Source: three-view drawing plus pictorial views. Frame: mm from the lowest corner of the part. Coordinates: 2 decimals unless noted, no trailing zeros. Write each loop counter-clockwise with the first axis right and the second up, starting at its lowest first coordinate (ties: lowest second). Pieces come first, ordered by that corner, then holes. Notation, with made-up numbers: (76, -0.5) - (91, -0.5) arc R25 cw to (91, 19.5) - close; hole circle Ø5 at (67, -25.5). An arc over 180 degrees is marked (long way). Answer as a JSON object with one key per item and string values. Group by question number.
Item 1: Section D-D on x = 30.5. Return loops of the section in (y, z), and give its area (3 significant figures).
Item 2: Section C-C on y = 82.5. Return loops of the section in (x, z), and give its area (3 significant figures).
Item 3: Line query: line 1 along Y through (x, z) = (25, 1.65); line 2 along X through (y, z) = (15.5, 1.05); line 3 along X through (y, z) = (81, 2). Output: solid intervals per line, ascending. Write a range as from..to.
Item 4: Section B-B on z = 1.4. Return loops of the section in (x, y), and give its area (3 significant figures).
Item 5: First-contact query: pin 1 Ø3 at (x, y) = (38, 33) entering from -Z; pin 2 Ø1.5 at (y, z) = (86.5, 1) entering from -X; pin 3 Ø1 at (x, z) = (21.5, 3.5) entering from +Y; pin 4 Ø1.3 at (x, z) = (20.5, 1.5) entering from -Y. Flat tips, straight axial feed; report the tip coordinate or a pass-through.
Item 6: Section A-A on x = 25. Return loops of the section in (y, z).
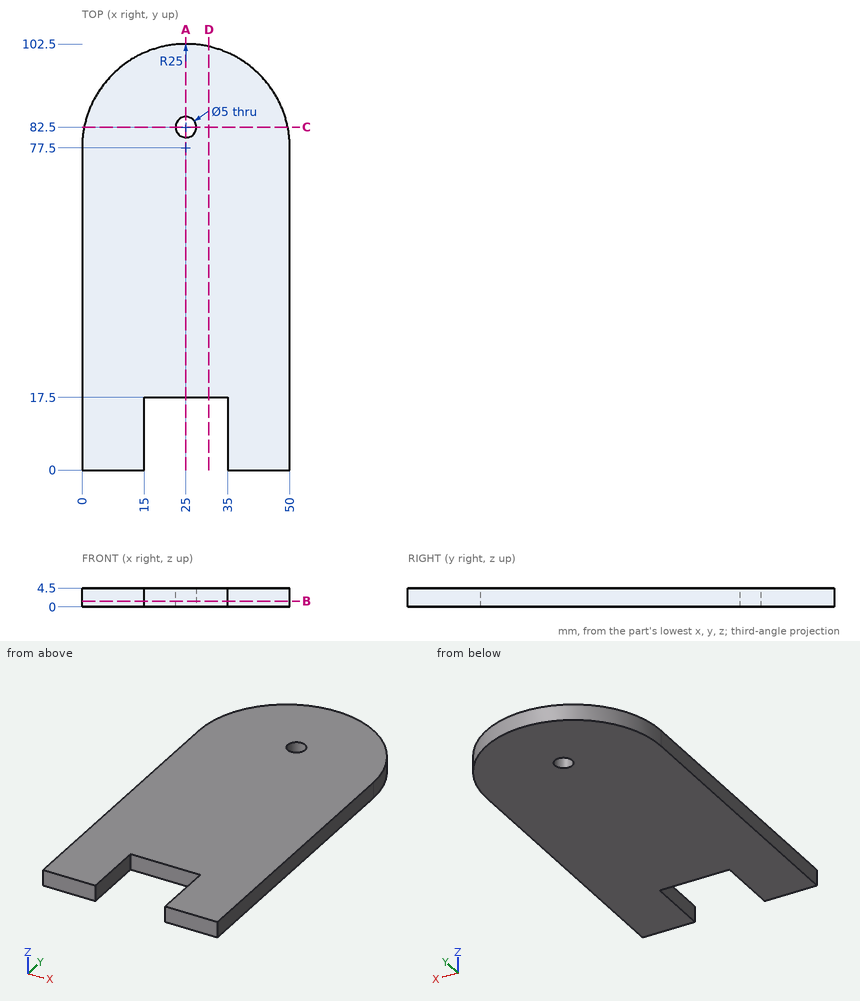
Checks:
{
 "1": {"outline": "(17.5, 0) - (101.89, 0) - (101.89, 4.5) - (17.5, 4.5) - close", "area": "380 mm^2"},
 "2": {"outline": "(0.51, 0) - (22.5, 0) - (22.5, 4.5) - (0.51, 4.5) - close; (27.5, 0) - (49.49, 0) - (49.49, 4.5) - (27.5, 4.5) - close", "area": "198 mm^2"},
 "3": {"line 1": "17.5..80, 85..102.5", "line 2": "0..15, 35..50", "line 3": "0.25..23, 27..49.75"},
 "4": {"outline": "(0, 0) - (15, 0) - (15, 17.5) - (35, 17.5) - (35, 0) - (50, 0) - (50, 77.5) arc R25 ccw to (0, 77.5) - close; hole circle Ø5 at (25, 82.5)", "area": "4,490 mm^2"},
 "5": {"pin 1": "z = 0", "pin 2": "x = 1.4", "pin 3": "y = 102.32", "pin 4": "y = 17.5"},
 "6": {"outline": "(17.5, 0) - (80, 0) - (80, 4.5) - (17.5, 4.5) - close; (85, 0) - (102.5, 0) - (102.5, 4.5) - (85, 4.5) - close"}
}
